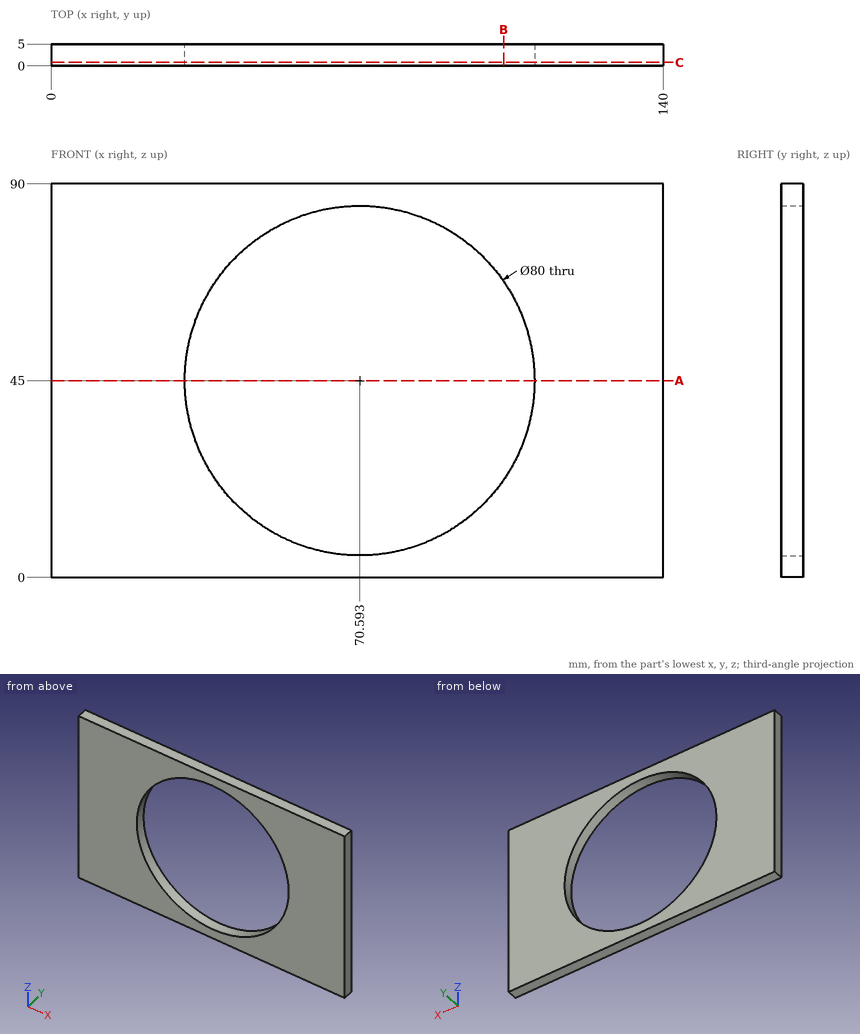
Answer from the drawing. Dimensions are ordinates in mm from the lowest x, y and z of the part. Give positions to 0.01 mm unless a question says otherwise; leave off trailing zeros. Write each loop counter-clockwise with the first axis right and the second up, starting at its lowest first coordinate (ties: lowest second). Pieces come first, ordered by that corner, then holes.
1) Find the intervals of material crossed by L1, parallel to X at y = 2.95, z = 45; L2, parallel to Z at x = 50.5, y = 1.4; L3, parallel to Z at x = 102, y = 4.75, in increasing order.
2) Section B-B (x = 103.5) is taken. Write down the section's boundary in (y, z).
3) Section C-C (y = 0.8) is taken. Write down the section's boundary in (x, z).
4) Section A-A (z = 45) is taken. Write down the section's boundary in (x, y).
Response:
1. L1: x = 0 to 30.59, 110.59 to 140
1. L2: z = 0 to 10.41, 79.59 to 90
1. L3: z = 0 to 20.23, 69.77 to 90
2. outline: (0, 0) - (5, 0) - (5, 22.26) - (0, 22.26) - close; (0, 67.74) - (5, 67.74) - (5, 90) - (0, 90) - close
3. outline: (0, 0) - (140, 0) - (140, 90) - (0, 90) - close; hole circle Ø80 at (70.59, 45)
4. outline: (0, 0) - (30.59, 0) - (30.59, 5) - (0, 5) - close; (110.59, 0) - (140, 0) - (140, 5) - (110.59, 5) - close
